Here's how the part is built. I have some questions about the finished solid (model axes, mm). Give positions to 0.01 mm unless a question says otherwise; leave off trailing zeros. Loops run counter-clockwise (first coordinate to the right, second up) from the corner with the lowest first, then second, coordinate; pieces in that order, holes last.
Q1. I need wall thicknesses on probe 1 along X at (y, z) = (3.65, -10); probe 2 along X at (y, z) = (1.25, -10); probe 3 along Z at (x, y) = (39, 3.75). Which ranges of each line are inside material? Lowest first, please.
Q2. Suppose I cut it at D-D (z = -7). List the corners of the cut face in (x, y) for me.
Q3. Suppose I cut it at C-C (y = 11). List the corners of the cut face in (x, z) for me.
Q4. Suppose I cut it at A-A (x = 9). List the corners of the cut face in (y, z) for me, and give its area (3 significant figures).
Q5. I'm going to push flat-ended pins straight in: P1, Ø2, axis at x = 25.5, y = 6.5, coming from the -Z side; P2, Ø9, axis at x = 39.5, z = -11, coming from the +Y side; P3, Ø5, axis at x = 13.5, y = 8.5, coming from the +Z side. Where does each tip first touch, or does it pass through?
Q6. Suppose I cut it at B-B (y = 2). List the corners of the cut face in (x, z) for me, and give its area (3 significant figures).
```python
from build123d import *

# Parameters (mm, degrees)
SKETCH1_R           = 2
BOSS_EXTRUDE1_DEPTH = 5
SKETCH2_R           = 4
CUT_EXTRUDE1_DEPTH  = 2
SKETCH3_R           = 2
BOSS_EXTRUDE2_DEPTH = 12
SKETCH4_W           = 51.589864231
SKETCH4_H           = 45.63525298
CUT_EXTRUDE2_DEPTH  = 5


with BuildPart() as part:
    # Sketch1 → Boss-Extrude1 (new body)
    with BuildSketch(Plane(origin=(0, 0, 0), x_dir=(1, 0, 0), z_dir=(0, 1, 0))):
        Polygon((0, 34), (0, 0), (49, 0), (49, 49), (15, 49), (15, 34), align=None)
        with Locations((9, 10)):
            Circle(SKETCH1_R, mode=Mode.SUBTRACT)
        with Locations((24, 18.03)):
            Circle(SKETCH1_R, mode=Mode.SUBTRACT)
        with Locations((39, 10)):
            Circle(SKETCH1_R, mode=Mode.SUBTRACT)
    extrude(amount=BOSS_EXTRUDE1_DEPTH)

    # Sketch2 → Cut-Extrude1 (cut)
    with BuildSketch(Plane(origin=(0, 5, 0), x_dir=(1, 0, 0), z_dir=(0, 1, 0))):
        with Locations((39, 10)):
            Circle(SKETCH2_R)
    extrude(amount=-CUT_EXTRUDE1_DEPTH, mode=Mode.SUBTRACT)

    # Sketch3 → Boss-Extrude2 (add)
    with BuildSketch(Plane(origin=(0, 5, 0), x_dir=(1, 0, 0), z_dir=(0, 1, 0))):
        with BuildLine():
            Line((15, 34), (0, 34))
            Line((0, 34), (0, 12.373527554))
            Line((0, 12.373527554), (0.318619525, 12.373527554))
            ThreePointArc((0.318619525, 12.373527554), (7.991284246, 18.943293159), (16.934577194, 14.247644612))
            ThreePointArc((16.934577194, 14.247644612), (16.486188802, 20.817302098), (21.110631854, 25.505156415))
            Line((21.110631854, 25.505156415), (21.110631854, 34))
            Line((21.110631854, 34), (15, 34))
        make_face()
        with BuildLine():
            Line((21.110631854, 12.373527554), (21.110631854, 25.505156415))
            ThreePointArc((21.110631854, 25.505156415), (16.486188802, 20.817302098), (16.934577194, 14.247644612))
            ThreePointArc((16.934577194, 14.247644612), (17.560142752, 13.25981653), (18.322788434, 12.373527554))
            Line((18.322788434, 12.373527554), (21.110631854, 12.373527554))
        make_face()
        with BuildLine():
            ThreePointArc((16.934577194, 14.247644612), (7.991284246, 18.943293159), (0.318619525, 12.373527554))
            Line((0.318619525, 12.373527554), (17.681380475, 12.373527554))
            ThreePointArc((17.681380475, 12.373527554), (17.360657331, 13.331577554), (16.934577194, 14.247644612))
        make_face()
        with BuildLine():
            ThreePointArc((32.014138239, 18.03), (28.531590006, 24.639924638), (21.110631854, 25.505156415))
            Line((21.110631854, 25.505156415), (21.110631854, 12.373527554))
            Line((21.110631854, 12.373527554), (18.322788434, 12.373527554))
            ThreePointArc((18.322788434, 12.373527554), (27.060102401, 10.623098826), (32.014138239, 18.03))
        make_face()
        with Locations((24, 18.03)):
            Circle(SKETCH3_R, mode=Mode.SUBTRACT)
        with BuildLine():
            Line((17.681380475, 12.373527554), (0.318619525, 12.373527554))
            ThreePointArc((0.318619525, 12.373527554), (0.08001053, 11.197408812), (0, 10))
            ThreePointArc((0, 10), (9, 1), (18, 10))
            ThreePointArc((18, 10), (17.91998947, 11.197408812), (17.681380475, 12.373527554))
        make_face()
        with Locations((9, 10)):
            Circle(SKETCH3_R, mode=Mode.SUBTRACT)
    extrude(amount=BOSS_EXTRUDE2_DEPTH)

    # Sketch4 → Cut-Extrude2 (cut)
    with BuildSketch(Plane(origin=(0, 17, 0), x_dir=(1, 0, 0), z_dir=(0, 1, 0))):
        with Locations((25.794932115, 11.18237351)):
            Rectangle(SKETCH4_W, SKETCH4_H)
    extrude(amount=-CUT_EXTRUDE2_DEPTH, mode=Mode.SUBTRACT)


solid = part.part
```
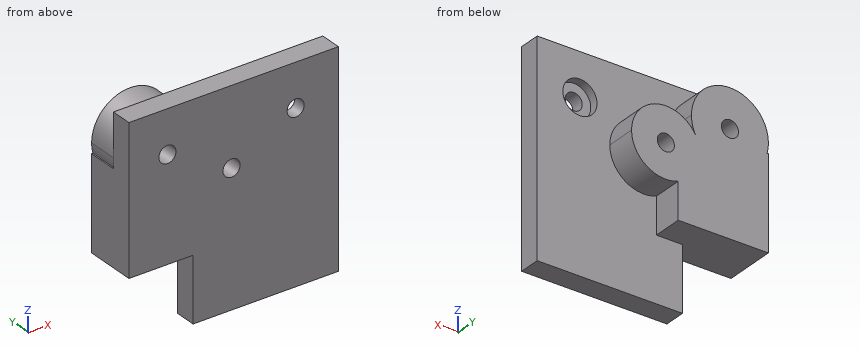
Solutions:
1. probe 1: x = 0 to 7, 11 to 35, 43 to 49
1. probe 2: x = 0 to 7, 11 to 37, 41 to 49
1. probe 3: z = -49 to -14, -6 to 0
2. outline: (0, 0) - (49, 0) - (49, 5) - (41.65, 5) - (41.65, 3) - (36.35, 3) - (36.35, 5) - (17.49, 5) - (17.49, 12) - (0.51, 12) - (0.51, 5) - (0, 5) - close
3. outline: (0, -34) - (21.11, -34) - (21.11, -25.51) arc R8.01 ccw (long way) to (16.93, -14.25) arc R9 ccw (long way) to (0.32, -12.37) - (0, -12.37) - close; hole circle Ø4 at (9, -10); hole circle Ø4 at (24, -18.03)
4. outline: (0, -34) - (12, -34) - (12, -12) - (0, -12) - close; (0, -8) - (12, -8) - (12, -1) - (5, -1) - (5, 0) - (0, 0) - close
4. area: 353 mm2
5. P1: stops at z = -26.03
5. P2: stops at y = 5
5. P3: stops at z = -1.23
6. outline: (0, -34) - (15, -34) - (15, -49) - (49, -49) - (49, 0) - (0, 0) - close; hole circle Ø4 at (9, -10); hole circle Ø4 at (24, -18.03); hole circle Ø4 at (39, -10)
6. area: 2,140 mm2
